Input: dimensioned drawing with shaded views. Units: mm. Origin: part minimum x, y, z. A direction names the side the tool comes from. Round coordinates to 2 decimals unless told otherwise and drop trailing zeros. Loops run counter-clockwise (first coordinate to the right, second up) from the corner with the lowest first, then second, coordinate; pieces in that order, holes last. Notation, with made-up numbers: M 1,40.25 L 39,40.25 A19 cw 39,67.25 Z; hole C 40,-21 d7. An arc over 180 degrees is marked long. Use one line per item in the form item = value. Start each with the question number.
Q1. Section query A-A, the plane y = 27. Output: boundary loops of the cut face in (x, z) (1 decimal).
Q2. First-contact query: P1, Ø5, axis at x = 78, y = 11.5, coming from the +Z side; P2, Ø3, axis at x = 93.5, z = 32.5, coming from the +Y side; P3, Ø10, axis at y = 9.5, z = 59.5, coming from the -X side; P4, Ø5, axis at x = 69.5, y = 49.5, coming from the +Z side. Flat tips, straight axial feed; report the tip coordinate or a pass-through.
Q3. Access query for the marked faces 1, 2, 3 and 4. Directions: +Z, -Z, +X, -X, +Y, -Y. A direction counts if a zero-diameter tool reaches every point of the face in a straight line with its end or side. Return the directions, or none.
Q4. Section query C-C, the plane z = 20.5. Output: boundary loops of the cut face in (x, y) (1 decimal), and give its area (3 significant figures).
Q5. Section query D-D, the plane x = 84. Output: boundary loops of the cut face in (y, z), and give its area (4 significant figures).
Q6. Section query B-B, the plane x = 109.5. Output: boundary loops of the cut face in (y, z) (1 decimal), and give its area (3 significant figures).
Q7. Ray query, line 1 along Y through (x, z) = (144.5, 64.5); line 2 along Z through (x, y) = (121, 55.5) (1 decimal); line 3 along Z through (x, y) = (60, 19). Return the intervals inside material, ascending.
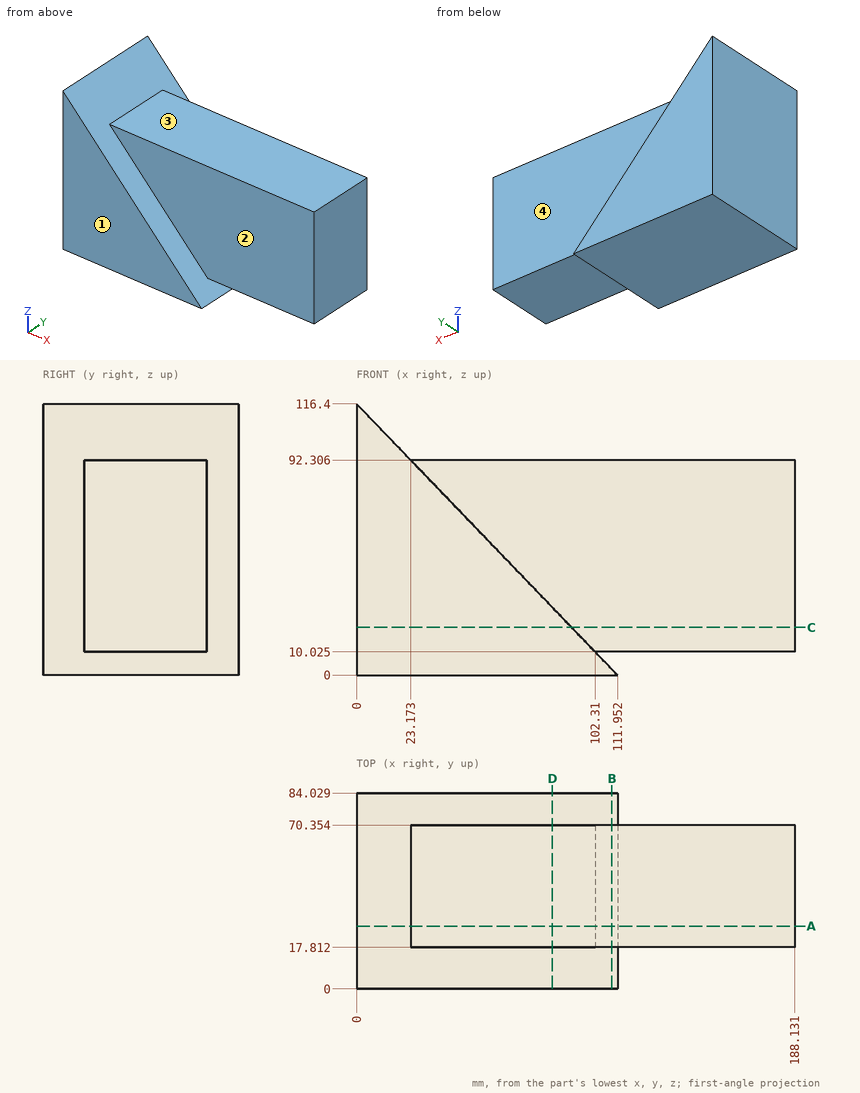
Results found:
q1.outline = M 0,0 L 112,0 L 102.3,10 L 188.1,10 L 188.1,92.3 L 23.2,92.3 L 0,116.4 Z
q2.P1 = 37.9
q2.P2 = 70.35
q2.P3 = 0
q2.P4 = 92.31
q3.face_1 = +Z, -Z, +X, -X, -Y
q3.face_2 = +Z, +X, -Y
q3.face_3 = +Z, +X, +Y, -Y
q3.face_4 = +Z, +X, +Y
q4.outline = M 0,0 L 92.2,0 L 92.2,17.8 L 188.1,17.8 L 188.1,70.4 L 92.2,70.4 L 92.2,84 L 0,84 Z
q4.area = 12,800 mm²
q5.outline = M 0,0 L 84.03,0 L 84.03,29.06 L 70.35,29.06 L 70.35,92.31 L 17.81,92.31 L 17.81,29.06 L 0,29.06 Z
q5.area = 5,765 mm²
q6.outline = M 0,0 L 84,0 L 84,2.5 L 0,2.5 Z; M 17.8,10 L 70.4,10 L 70.4,92.3 L 17.8,92.3 Z
q6.area = 4,540 mm²
q7.line_1 = 17.81 to 70.35
q7.line_2 = 10 to 92.3
q7.line_3 = 0 to 92.31
